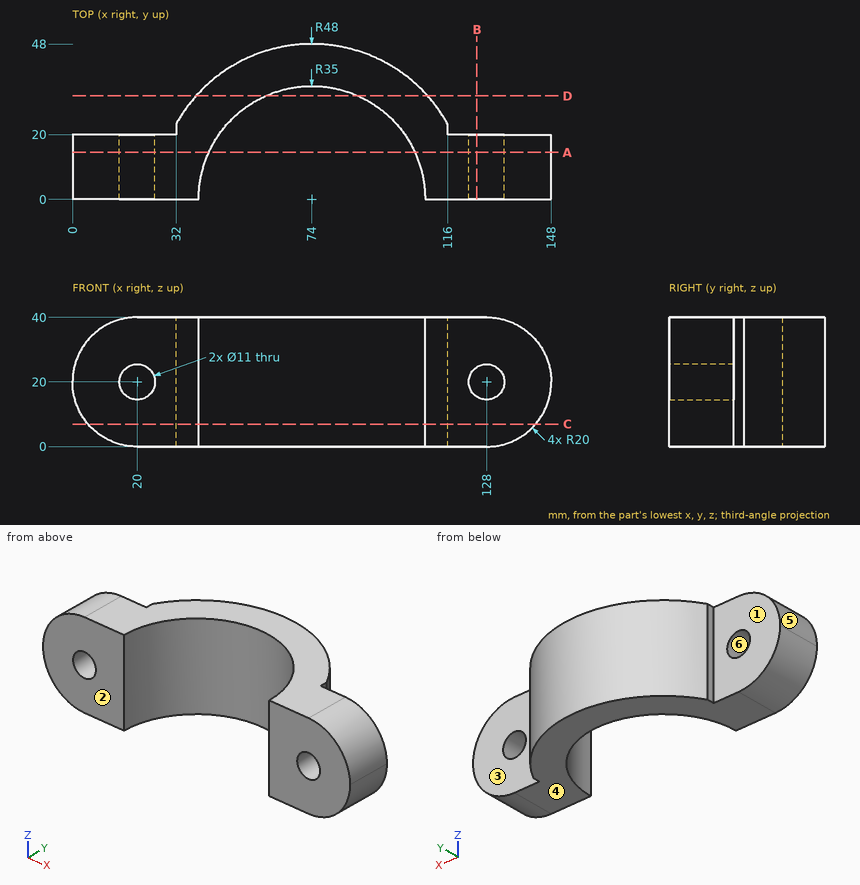
Design review of the part shown in the three views and the two pictorial views. Dimensions are in mm from the part's minimum x, y and z. A direction names the side the tool comes from. Give positions to 0.01 mm unless a question says otherwise; leave off trailing zeros. Loops run counter-clockwise (first coordinate to the right, second up) from the corner with the lowest first, then second, coordinate; pieces in that order, holes last. Notation, with made-up numbers: (54, 86) -> (83, 86) arc R33 ccw to (83, 125) -> close; hole circle Ø6 at (55, 72.25). An arc over 180 degrees is marked (long way). Write each question's results on one line, items separated by ' | '.
Q1. Take a section at D-D, the plane y = 32. Write out the cut boundary in (x, z).
Reply:
outline: (38.22, 0) -> (59.82, 0) -> (59.82, 40) -> (38.22, 40) -> close; (88.18, 0) -> (109.78, 0) -> (109.78, 40) -> (88.18, 40) -> close
Q2. Take a section at B-B, the plane x = 125. Write out the cut boundary in (y, z), plus the area to 3 significant figures.
Reply:
outline: (0, 0) -> (20, 0) -> (20, 15.39) -> (0, 15.39) -> close; (0, 24.61) -> (20, 24.61) -> (20, 40) -> (0, 40) -> close | area: 616 mm²
Q3. The part is to be moulded in two halves that separate along Z. For the marked faces 3, 4, 5 and 6, say which applies: +Z half, -Z half, draft (parallel to the pull), parting line (faces both ways), or undercut.
Reply:
face 3: draft | face 4: -Z half | face 5: +Z half | face 6: undercut
Q4. Machinability: for the marked faces 1 and 2, which of the approach directions +Z, -Z, +X, -X, +Y, -Y give a long, thin tool a straight path to every point of the face, cutting with its end or side? Answer none if there is none.
Reply:
face 1: +Z, -Z, -X, +Y | face 2: +Z, -Z, +X, -X, -Y
Q5. Take a section at C-C, the plane z = 7. Write out the cut boundary in (x, y), plus the area to 3 significant figures.
Reply:
outline: (4.8, 0) -> (39, 0) arc R35 cw to (109, 0) -> (143.2, 0) -> (143.2, 20) -> (116, 20) -> (116, 23.24) arc R48 ccw to (32, 23.24) -> (32, 20) -> (4.8, 20) -> close | area: 2,590 mm²
Q6. Wall thickness on L1, parallel to X at y = 4, z = 20; L2, parallel to X at y = 6.75, z = 20; L3, parallel to Y at x = 134, z = 9: over which ranges is each line inside the solid? List them lowest first.
Reply:
L1: x = 0 to 14.5, 25.5 to 39.23, 108.77 to 122.5, 133.5 to 148 | L2: x = 0 to 14.5, 25.5 to 39.66, 108.34 to 122.5, 133.5 to 148 | L3: y = 0 to 20
Q7. For pin 1 Ø12 at (x, y) = (96.5, 11.5) entering from -Z; pin 2 Ø2 at (y, z) = (41.5, 19.5) entering from +X; pin 3 Ø2.5 at (y, z) = (21.5, 14.5) entering from +X; pin 4 Ø5 at (x, z) = (28.5, 34.5) entering from +Y, all flat-tipped, find the tip position at first contact; note any pin that passes through.
Reply:
pin 1: passes through | pin 2: stops at x = 99.76 | pin 3: stops at x = 116 | pin 4: stops at y = 20
Q8. Take a section at A-A, the plane y = 14.5. Give the number of separate pieces and of enclosed holes in the cut face, plus the area to 3 significant figures.
Reply:
separate pieces: 2 | enclosed holes: 2 | area: 2,840 mm²
